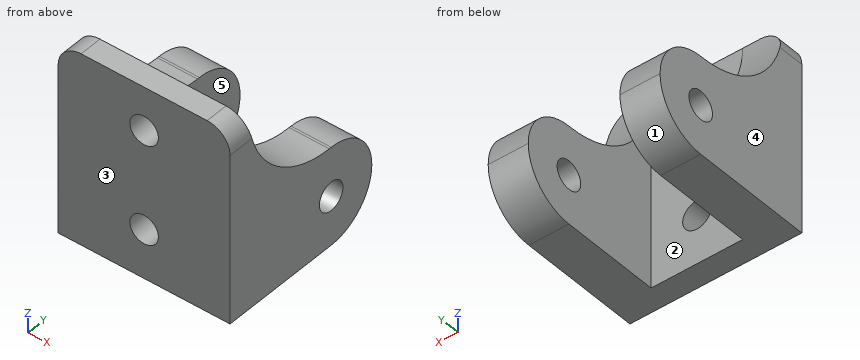
```python
from build123d import *

# Parameters (mm, degrees)
SKETCH1_W                            = 38.1
SKETCH1_H                            = 42.672
BOSS_EXTRUDE1_DEPTH                  = 5.08
SKETCH2_W                            = 8.89
SKETCH2_H                            = 21.844
BOSS_EXTRUDE2_DEPTH                  = 33.02
FILLET1_R                            = 10.922
FILLET2_R                            = 21.59
FILLET3_R                            = 5.08
F_1_1_DIAMETER_HOLE1_D               = 6.35
F_1_1_DIAMETER_HOLE1_DEPTH           = 50.8
F_1_1_DIAMETER_HOLE1_TIP             = 1.907732465
F_1_1_DIAMETER_HOLE1_ON_FACE_2_D     = 6.35
F_1_1_DIAMETER_HOLE1_ON_FACE_2_DEPTH = 50.8
F_1_1_DIAMETER_HOLE1_ON_FACE_2_TIP   = 1.907732465


# Some blends are built 0.0001 mm under size
with BuildPart() as part:
    # Sketch1 → Boss-Extrude1 (new body)
    with BuildSketch(Plane(origin=(0, 0, 0), x_dir=(1, 0, 0), z_dir=(0, 1, 0))):
        with Locations((1.652063174, -2.269767862)):
            Rectangle(SKETCH1_W, SKETCH1_H)
    extrude(amount=BOSS_EXTRUDE1_DEPTH)

    # Sketch2 → Boss-Extrude2 (add)
    with BuildSketch(Plane(origin=(0, 5.08, 0), x_dir=(1, 0, 0), z_dir=(0, 1, 0))):
        with Locations((16.257063174, 8.144232138)):
            Rectangle(SKETCH2_W, SKETCH2_H)
        with Locations((-12.952936826, 8.144232138)):
            Rectangle(SKETCH2_W, SKETCH2_H)
    extrude(amount=BOSS_EXTRUDE2_DEPTH)

    # Fillet1
    fillet1_edges = [part.edges().sort_by_distance(p)[0] for p in [
        (-12.952936826, 38.1, -19.066232138),
        (16.257063174, 38.1, -19.066232138),
        (16.257063174, 38.1, 2.777767862),
        (-12.952936826, 38.1, 2.777767862),
    ]]
    fillet(fillet1_edges, radius=FILLET1_R - 0.0001)  # a hair under: the kernel refuses the full size

    # Fillet2
    # the kernel refuses this fillet: 21.59 mm, written as the material it adds along each edge
    with BuildSketch(Plane(origin=(-42.129308703, 5.08, 2.777767862), x_dir=(0, 0, 1), z_dir=(1, 0, 0))) as fillet2_piece_1_section:
        with BuildLine():
            CenterArc((21.59, -21.576548751), FILLET2_R, 92.022624053, 87.977375947)
            Line((0, -21.576548751), (-0.4318, -21.576548751))
            Line((-0.4318, -21.576548751), (-0.4318, 0))
            Line((-0.4318, 0), (0, 0.4318))
            ThreePointArc((0, 0.4318), (10.414, 0.4318), (20.81276, 0.431530975))
            Line((20.81276, 0.431530975), (20.828, 0))
        make_face()
    fillet2_piece_1 = extrude(amount=62.831371877, mode=Mode.PRIVATE)
    fillet2_piece_1 = split(fillet2_piece_1, bisect_by=Plane(origin=(-17.397936826, 9.985892861, 7.610379984), z_dir=(1, 0, 0)), keep=Keep.TOP, mode=Mode.PRIVATE)
    fillet2_piece_1 = split(fillet2_piece_1, bisect_by=Plane(origin=(-8.507936826, 9.985892861, 7.610379984), z_dir=(-1, 0, 0)), keep=Keep.TOP, mode=Mode.PRIVATE)
    add(fillet2_piece_1)
    with BuildSketch(Plane(origin=(11.812063174, 5.08, 2.777767862), x_dir=(0, 0, 1), z_dir=(1, 0, 0))) as fillet2_piece_2:
        with BuildLine():
            CenterArc((21.59, -21.576548751), FILLET2_R, 92.022624053, 87.977375947)
            Line((0, -21.576548751), (-0.4318, -21.576548751))
            Line((-0.4318, -21.576548751), (-0.4318, 0))
            Line((-0.4318, 0), (0, 0.4318))
            ThreePointArc((0, 0.4318), (10.414, 0.4318), (20.81276, 0.431530975))
            Line((20.81276, 0.431530975), (20.828, 0))
        make_face()
    extrude(amount=8.89)
    with BuildSketch(Plane(origin=(45.433435051, 5.08, 2.777767862), x_dir=(0, 0, 1), z_dir=(-1, 0, 0))) as fillet2_piece_3_section:
        with BuildLine():
            CenterArc((21.59, 21.576548751), FILLET2_R, 180, 87.977375947)
            Line((0, 21.576548751), (-0.4318, 21.576548751))
            Line((-0.4318, 21.576548751), (-0.4318, 0))
            Line((-0.4318, 0), (0, -0.4318))
            ThreePointArc((0, -0.4318), (10.414, -0.4318), (20.81276, -0.431530975))
            Line((20.81276, -0.431530975), (20.828, 0))
        make_face()
    fillet2_piece_3 = extrude(amount=62.831371877, mode=Mode.PRIVATE)
    fillet2_piece_3 = split(fillet2_piece_3, bisect_by=Plane(origin=(20.702063174, 9.985892861, 7.610379984), z_dir=(-1, 0, 0)), keep=Keep.TOP, mode=Mode.PRIVATE)
    fillet2_piece_3 = split(fillet2_piece_3, bisect_by=Plane(origin=(11.812063174, 9.985892861, 7.610379984), z_dir=(1, 0, 0)), keep=Keep.TOP, mode=Mode.PRIVATE)
    add(fillet2_piece_3)
    with BuildSketch(Plane(origin=(-8.507936826, 5.08, 2.777767862), x_dir=(0, 0, 1), z_dir=(-1, 0, 0))) as fillet2_piece_4:
        with BuildLine():
            CenterArc((21.59, 21.576548751), FILLET2_R, 180, 87.977375947)
            Line((0, 21.576548751), (-0.4318, 21.576548751))
            Line((-0.4318, 21.576548751), (-0.4318, 0))
            Line((-0.4318, 0), (0, -0.4318))
            ThreePointArc((0, -0.4318), (10.414, -0.4318), (20.81276, -0.431530975))
            Line((20.81276, -0.431530975), (20.828, 0))
        make_face()
    extrude(amount=8.89)

    # Fillet3
    fillet3_edges = [part.edges().sort_by_distance(p)[0] for p in [
        (20.702063174, 2.54, 23.605767862),
        (-17.397936826, 2.54, 23.605767862),
    ]]
    fillet(fillet3_edges, radius=FILLET3_R)

    # 1 (1) Diameter Hole1
    with Locations(Plane(origin=(1.652063174, 5.08, 13.953767862), x_dir=(0, 0, 1), z_dir=(0, 1, 0))):
        with Locations((0, 0), (-22.098, 0)):
            Hole(F_1_1_DIAMETER_HOLE1_D / 2, depth=F_1_1_DIAMETER_HOLE1_DEPTH)
            with Locations((0, 0, -(F_1_1_DIAMETER_HOLE1_DEPTH + F_1_1_DIAMETER_HOLE1_TIP / 2))):  # 118° drill point
                Cone(0, F_1_1_DIAMETER_HOLE1_D / 2, F_1_1_DIAMETER_HOLE1_TIP, mode=Mode.SUBTRACT)

    # 1 (1) Diameter Hole1 on face 2
    with Locations(Plane(origin=(20.702063174, 27.178, -8.144232138), x_dir=(0, 0, 1), z_dir=(1, 0, 0))):
        with Locations((0, 0)):
            Hole(F_1_1_DIAMETER_HOLE1_ON_FACE_2_D / 2, depth=F_1_1_DIAMETER_HOLE1_ON_FACE_2_DEPTH)
            with Locations((0, 0, -(F_1_1_DIAMETER_HOLE1_ON_FACE_2_DEPTH + F_1_1_DIAMETER_HOLE1_ON_FACE_2_TIP / 2))):  # 118° drill point
                Cone(0, F_1_1_DIAMETER_HOLE1_ON_FACE_2_D / 2, F_1_1_DIAMETER_HOLE1_ON_FACE_2_TIP, mode=Mode.SUBTRACT)


solid = part.part
```
Read the model definition and answer for the solid it produces. Units are mm, in the model's axes. Face numbers are marked on the shaded views. A direction names the side the tool comes from. Coordinates: 2 decimals unless noted, no trailing zeros. Order: outer loops, then holes, each group sorted by start corner. A loop starts at its lowest first (then second) coordinate and runs counter-clockwise, first axis right, second up. Notation, with made-up numbers: (-4, 8) - (29, 8) arc R16 cw to (29, 13) - close; hole circle Ø2 at (41.25, -6). An arc over 180 degrees is marked (long way). Answer as a JSON object with one key per item and string values. Group by question number.
Item 1: Section A-A (y = 35) is taken. Give the vertices of the cut face in (x, z).
Item 2: The mould has two halves that part along X. Classify the marked faces 3, 4 and 5: +X half, -X half, draft (parallel to the pull), parting line (faces both ways), or undercut.
Item 3: Flat-ended cylindrical pins translate along their axes: P1, Ø1, axis at x = 13, y = 22.5, coming from the +Z side; P2, Ø5, axis at x = -4.5, z = -5, coming from the -Y side; P3, Ø5, axis at x = 12.5, z = -13.5, coming from the +Y side; P4, Ø3, axis at x = 4.5, z = 0, coming from the +Y side. Find the tip coordinate at first contact, or state that the pin passes through.
Item 4: Section D-D (z = 13) is taken. Give the vertices of the cut face in (x, y).
Item 5: Section C-C (x = 2.5) is taken. Give the vertices of the cut face in (y, z).
Item 6: Consider probe 1 along X at (y, z) = (10.5, 5); probe 2 along Y at (x, z) = (-6.5, 19); probe 3 along Z at (x, y) = (18.5, 17.5). Determine where each line is inside the solid, lowest interval first. Write a range as from..to.
Item 7: A tool of negligible diameter and unlimited length cuts with its end or side. For the marked faces 1 and 2, from which of +Z, -Z, +X, -X, +Y, -Y can it reach the whole face along a straight path? Write none if from no direction.
Results are:
{
 "1": {"outline": "(-17.4, -15.77) - (-8.51, -15.77) - (-8.51, -0.52) - (-17.4, -0.52) - close; (11.81, -15.77) - (20.7, -15.77) - (20.7, -0.52) - (11.81, -0.52) - close"},
 "2": {"face 3": "draft", "face 4": "-X half", "face 5": "undercut"},
 "3": {"P1": "stops at z = 3.29", "P2": "stops at y = 0", "P3": "stops at y = 37.72", "P4": "stops at y = 5.08"},
 "4": {"outline": "(-17.4, 0) - (-1.38, 0) - (-1.38, 5.08) - (-8.51, 5.08) - (-8.51, 8.3) - (-17.4, 8.3) - close; (4.68, 0) - (20.7, 0) - (20.7, 8.3) - (11.81, 8.3) - (11.81, 5.08) - (4.68, 5.08) - close"},
 "5": {"outline": "(0, -19.07) - (5.08, -19.07) - (5.08, -11.2) - (0, -11.2) - close; (0, -5.08) - (5.08, -5.08) - (5.08, 10.89) - (0, 10.89) - close; (0, 17.01) - (5.08, 17.01) - (5.08, 23.61) - (0, 23.61) - close"},
 "6": {"probe 1": "x = -17.4..-8.51, 11.81..20.7", "probe 2": "y = 0..5.08", "probe 3": "z = -19.07..4.82"},
 "7": {"face 1": "-Z, +X, -X, +Y", "face 2": "+Z, -Z, +Y"}
}
